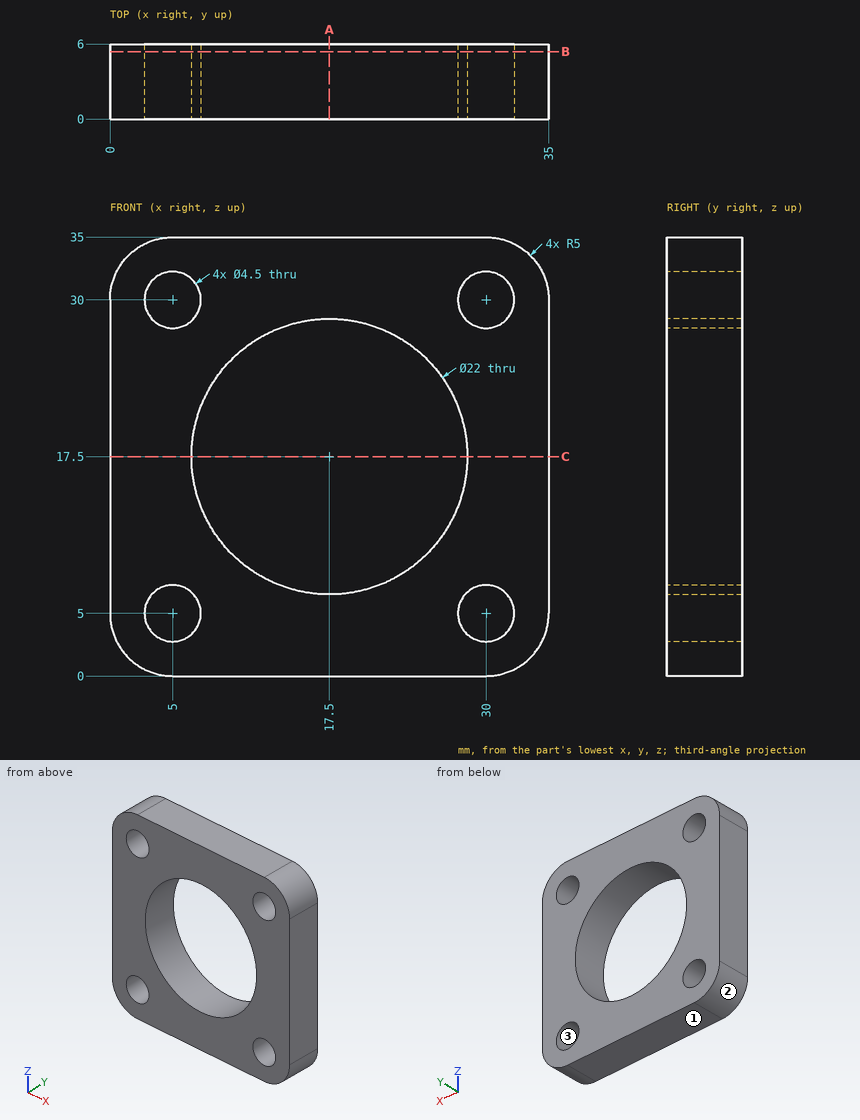
The figure shows three views and two pictorial views of one solid part (mm, origin at its lowest corner). Answer the questions. Give positions to 0.01 mm unless a question says otherwise; leave off trailing zeros. Write each loop counter-clockwise with the first axis right and the second up, starting at its lowest first coordinate (ties: lowest second). Pieces come first, ordered by that corner, then holes. Notation, with made-up numbers: (-18, -14) - (21, -14) arc R13 ccw to (21, 3) - close; hole circle Ø9 at (85, 70.5). An arc over 180 degrees is marked (long way). Use CSV: the item, a comma, the result in double quotes. Start each with the question number.
Item 1: Consider line 1 (Z direction, x = 5, y = 3.85); line 2 (X direction, y = 4.5, z = 17.5). Determine where each line is inside the solid, lowest interval first.
Item 2: The part is cut by section C-C, the plane z = 17.5. Give the vertices of the cut face in (x, y), and give its area (3 significant figures).
Item 3: The part is cut by section A-A, the plane x = 17.5. Give the vertices of the cut face in (y, z), and give its area (3 significant figures).
Item 4: The part is cut by section B-B, the plane y = 5.4. Give the vertices of the cut face in (x, z), and give its area (3 significant figures).
Item 5: The mould has two halves that part along X. Classify the marked faces 1, 2 and 3: pulls with the +X half, pulls with the -X half, needs draft (parallel to the pull), parting line crosses it, or undercut.
Taken from the geometry:
1,line 1,"0 to 2.75, 7.25 to 27.75, 32.25 to 35"
1,line 2,"0 to 6.5, 28.5 to 35"
2,outline,"(0, 0) - (6.5, 0) - (6.5, 6) - (0, 6) - close; (28.5, 0) - (35, 0) - (35, 6) - (28.5, 6) - close"
2,area,"78.0 mm2"
3,outline,"(0, 0) - (6, 0) - (6, 6.5) - (0, 6.5) - close; (0, 28.5) - (6, 28.5) - (6, 35) - (0, 35) - close"
3,area,"78.0 mm2"
4,outline,"(0, 5) arc R5 ccw to (5, 0) - (30, 0) arc R5 ccw to (35, 5) - (35, 30) arc R5 ccw to (30, 35) - (5, 35) arc R5 ccw to (0, 30) - close; hole circle Ø4.5 at (5, 5); hole circle Ø4.5 at (5, 30); hole circle Ø22 at (17.5, 17.5); hole circle Ø4.5 at (30, 5); hole circle Ø4.5 at (30, 30)"
4,area,"760 mm2"
5,face 1,"needs draft"
5,face 2,"pulls with the -X half"
5,face 3,"undercut"
